Autodesk Inventor part; units mm, degrees
ref_plane "РабПлоскость6" through (0, -10.8, 0) normal (1, 0, 0) x (0, 0, -1)
ref_plane "YZ Plane" through (0, 0, 0) normal (1, 0, 0) x (0, 1, 0)
ref_plane "XZ Plane" through (0, 0, 0) normal (0, 1, 0) x (-1, 0, 0)
sketch "Эскиз1" plane through (0, 0, 0) normal (0, 0, 1) x (1, 0, 0)
  circle A0 centre (0, 0) radius 5.75
  circle A1 centre (0, 0) radius 9.55
  line L0 (9.55, 13.5) -> (-9.55, 13.5)
  line L1 (-9.55, 13.5) -> (-9.55, 0)
  line L2 (-9.55, 0) -> (9.55, 0)
  line L3 (9.55, 0) -> (9.55, 13.5)
  line L4 (9.55, 0) -> (-9.55, 0)
  line L5 (-9.55, 0) -> (-9.55, -10.8)
  line L6 (-9.55, -10.8) -> (9.55, -10.8)
  line L7 (9.55, -10.8) -> (9.55, 0)
  point P0 (9.55, 0)
  point P1 (0, 9.55)
  point P2 (-9.55, 0)
  point P3 (9.55, 0)
  point P4 (-9.55, 0)
  dimension "d0" = 11.5
  dimension "d1" = 19.1
  dimension "d64" = 10.8
  dimension "d85" = 13.5
extrude "Выдавливание1" add sketch "Эскиз1" along normal blind 8 contours L2 A1 A0 | A0 L2 A1 | L7 L6 L5 A1 | A1 L1 L0 L3
sketch "Эскиз15" plane through (0, 0, 8) normal (0, 0, 1) x (1, 0, 0)
  circle A0 centre (0, 0) radius 5.75
  circle A1 centre (0, 0) radius 7.55
  dimension "d67" = 15.1
extrude "Выдавливание9" cut sketch "Эскиз15" against normal blind 4
ref_plane "РабПлоскость6" through (0, -10.8, 0) normal (1, 0, 0) x (0, 0, -1)
sketch "Эскиз16" plane through (-9.55, -10.8, 0) normal (0, -1, 0) x (1, 0, 0)
  line L0 (0, 8) -> (19.1, 8)
  line L1 (19.1, 8) -> (24.7, 8)
  line L2 (24.7, 8) -> (24.7, 0)
  line L3 (24.7, 0) -> (19.1, 0)
  line L4 (19.1, 0) -> (19.1, 8)
  point P0 (9.55, 0)
  dimension "d70" = 5.6
  dimension "d71" = 8
extrude "Выдавливание10" add sketch "Эскиз16" against normal up to surface (24.3 mm away)
sketch "Эскиз17" plane through (-9.55, 13.5, 0) normal (0, 1, 0) x (1, 0, 0)
  line L0 (24.7, 0) -> (24.7, -8)
  line L1 (24.7, -4) -> (20.15, -4)
  point P0 (9.55, 0)
  dimension "d82" = 4.55
hole "Отверстие4" at (10.6, 13.5, 4) direction (0, -1, 0) diameter 3.2 end through all
fillet "Сопряжение5" radius 5.05 1 edges at (15.15, 1.35, 8)
fillet "Сопряжение5" radius 2.95 1 edges at (15.15, 1.35, 0)
mirror "Зеркальное отражение5" about plane through (0, -10.8, 0) normal (1, 0, 0) of "Сопряжение5", "Отверстие4", "Выдавливание10"
ref_plane "РабПлоскость7" through (0, -10.8, 0) normal (1, 0, 0) x (0, 0, -1)
properties part number "Крепление дифференциала"
CAD build for the part. Positions are in the model's coordinates, mm. A direction names the side the tool comes from. Coordinates: 2 decimals unless noted, no trailing zeros. Order: outer loops, then holes, each group sorted by start corner. A loop starts at its lowest first (then second) coordinate and runs counter-clockwise, first axis right, second up. Notation, with made-up numbers: (34, 9) - (38, 9) arc R11 ccw to (38, 13) - close; hole circle Ø2 at (69.25, -34). An arc over 180 degrees is marked (long way). Answer in a Markdown table with one row per item.
1. Slice it at B-B, the plane x = -2. List the corners of the cut face in (y, z), then the cut area to 3 significant figures.
Answer:
| item | result |
|---|---|
| outline | (-10.8, 0) - (-5.39, 0) - (-5.39, 4) - (-7.28, 4) - (-7.28, 8) - (-10.8, 8) - close; (5.39, 0) - (13.5, 0) - (13.5, 8) - (7.28, 8) - (7.28, 4) - (5.39, 4) - close |
| area | 93.0 mm² |
2. 3-axis set-ups, long thin cutter, end or side, ignore diameter. For faces 1 (the face through (0, -10.8, 4)), 2 (the face through (-1.64, -7.37, 6.03)): which of +Z, -Z, +X, -X, +Y, -Y reach the whole face in a straight line?
Answer:
| item | result |
|---|---|
| face 1 | +Z, -Z, +X, -X, -Y |
| face 2 | +Z |
3. Pull direction Z, two halves, no side cores. Call faces 3 (the face through (-14.26, 1.52, 0.84)), 4 (the face through (12.16, 1.18, 3.65)), 5 (the face through (-0.75, -5.7, 1.97)): +Z half, -Z half, draft (parallel to the pull), parting line (faces both ways), or undercut.
Answer:
| item | result |
|---|---|
| face 3 | -Z half |
| face 4 | undercut |
| face 5 | draft |
4. Drill centre lines: L1, parallel to Y at x = 0, z = 2.65; L2, parallel to X at y = -4, z = 2.75; L3, parallel to Y at x = 0, z = 4.75. Where is each one in solid material? Low to high. Write a range as from..to.
Answer:
| item | result |
|---|---|
| L1 | -10.8..-5.75, 5.75..13.5 |
| L2 | -15.14..-11.6, -9.6..-4.13, 4.13..9.6, 11.6..15.14 |
| L3 | -10.8..-7.55, 7.55..13.5 |
5. Flat gauge pins, fed straight in: P1, Ø1.5, axis at y = -1, z = 2, coming from the +X side; P2, Ø1.9, axis at x = 10.6, z = 4, coming from the -Y side; P3, Ø3, axis at y = -3, z = 5, coming from the -X side; P4, Ø13, axis at x = 0, y = 0, coming from the +Z side. Where does each tip first touch, or does it go through?
Answer:
| item | result |
|---|---|
| P1 | x = 15.14 |
| P2 | through |
| P3 | x = -15.12 |
| P4 | z = 4 |
6. Slice it at A-A, the plane y = 9.75. Give the number of separate pieces and of enclosed holes in the cut face, then the cut area to 3 significant figures.
Answer:
| item | result |
|---|---|
| separate pieces | 1 |
| enclosed holes | 2 |
| area | 212 mm² |
7. Slice it at D-D, the plane x = 11. List the corners of the cut face in (y, z), then the cut area to 3 significant figures.
Answer:
| item | result |
|---|---|
| outline | (-10.8, 0) - (13.5, 0) - (13.5, 2.45) - (-10.8, 2.45) - close; (-10.8, 5.55) - (13.5, 5.55) - (13.5, 7.92) - (-10.8, 7.92) - close |
| area | 117 mm² |
